Read the model definition and answer for the solid it produces. Units are mm, in the model's axes. Give positions to 0.01 mm unless a question says otherwise; leave off trailing zeros. Write each loop counter-clockwise with the first axis right and the second up, starting at its lowest first coordinate (ties: lowest second). Pieces come first, ordered by that corner, then holes. Notation, with made-up numbers: M -39.75,61.5 L -5.75,61.5 A27 cw -5.75,97.5 Z; hole C -2,-14 d11. An arc over 180 degrees is marked long. Put each result on its own line as item: value.
from build123d import *

# Parameters (mm, degrees)
SKETCH1_R           = 2.54
SKETCH1_R_2         = 20.447
BOSS_EXTRUDE1_DEPTH = 1.3462


with BuildPart() as part:
    # Sketch1 → Boss-Extrude1 (new body)
    with BuildSketch(Plane.XY):
        with BuildLine():
            Line((48.387, 3.666174209), (48.387, 42.037))
            ThreePointArc((48.387, 42.037), (46.527128061, 46.527128061), (42.037, 48.387))
            Line((42.037, 48.387), (6.35, 48.387))
            ThreePointArc((6.35, 48.387), (1.859871939, 46.527128061), (0, 42.037))
            Line((0, 42.037), (0, 3.666174209))
            ThreePointArc((0, 3.666174209), (0.850738686, 0.491174209), (3.175, -1.833087105))
            Line((3.175, -1.833087105), (21.0185, -12.135036633))
            ThreePointArc((21.0185, -12.135036633), (24.1935, -12.985775319), (27.3685, -12.135036633))
            Line((27.3685, -12.135036633), (45.212, -1.833087105))
            ThreePointArc((45.212, -1.833087105), (47.536261314, 0.491174209), (48.387, 3.666174209))
        make_face()
        with Locations((6.35, 42.037)):
            Circle(SKETCH1_R, mode=Mode.SUBTRACT)
        with Locations((42.037, 42.037)):
            Circle(SKETCH1_R, mode=Mode.SUBTRACT)
        with Locations((42.037, 3.666174209)):
            Circle(SKETCH1_R, mode=Mode.SUBTRACT)
        with Locations((6.35, 3.666174209)):
            Circle(SKETCH1_R, mode=Mode.SUBTRACT)
        with Locations((24.1935, -6.635775319)):
            Circle(SKETCH1_R, mode=Mode.SUBTRACT)
        with Locations((24.1935, 24.1935)):
            Circle(SKETCH1_R_2, mode=Mode.SUBTRACT)
    extrude(amount=BOSS_EXTRUDE1_DEPTH)


solid = part.part
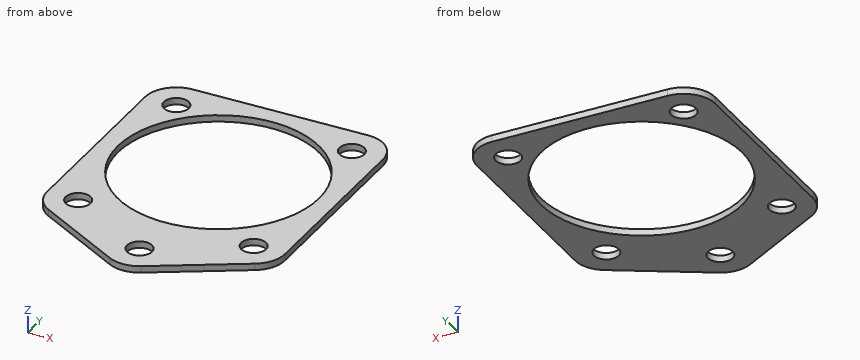
(1) Section C-C on x = 26 is taken. Determine the outline of the cut face in (y, z), and give its area (3 significant figures).
Result:
outline: M -12.72,0 L -8.42,0 L -8.42,1.35 L -12.72,1.35 Z; M -4.85,0 L 3.83,0 L 3.83,1.35 L -4.85,1.35 Z; M 44.56,0 L 48.39,0 L 48.39,1.35 L 44.56,1.35 Z
area: 22.6 mm²
(2) Section D-D on z = 1 is taken. Give the number of separate pieces and of enclosed holes in the cut face, and give its area (3 significant figures).
Result:
separate pieces: 1
enclosed holes: 6
area: 1,240 mm²
(3) Section A-A on y = 23.5 is taken. Determine the outline of the cut face in (x, z).
Result:
outline: M 0,0 L 3.76,0 L 3.76,1.35 L 0,1.35 Z; M 44.63,0 L 48.39,0 L 48.39,1.35 L 44.63,1.35 Z
(4) Section B-B on x = 17 is taken. Determine the outline of the cut face in (y, z).
Result:
outline: M -9.81,0 L 5.05,0 L 5.05,1.35 L -9.81,1.35 Z; M 43.33,0 L 48.39,0 L 48.39,1.35 L 43.33,1.35 Z
(5) Straight lines are drawn through the part: line 1 along X through (y, z) = (24, 0.6); line 2 along Y through (x, z) = (40.5, 0.4); line 3 along Y through (x, z) = (22, 0.4). For each, find the intervals that lie inside material, in ascending order. Write a range as from..to.
Result:
line 1: x = 0..3.75, 44.64..48.39
line 2: y = -4.55..1.64, 5.69..11.86, 36.53..40.01, 44.06..48.39
line 3: y = -12.59..-7.92, -5.36..3.86, 44.52..48.39
